The model under review builds one solid part; all positions refer to its coordinate system, in mm. Round coordinates to 2 decimals unless told otherwise and drop trailing zeros. Write each loop counter-clockwise with the first axis right and the second up, starting at its lowest first coordinate (ties: lowest second). Pieces come first, ordered by that corner, then holes. Notation, with made-up numbers: (49, -4.75) -> (59, -4.75) arc R13 ccw to (59, 12.25) -> close; hole circle Ø6 at (59.25, 44). An arc over 180 degrees is marked (long way). Return JSON: item names as keys, results as strings. Group by question number.
1. Take a section at A-A, the plane y = 0. Write out the cut boundary in (x, z), then the cut area to 3 significant figures.
2. For line 1 along Z through (x, y) = (7, 0); line 2 along Y through (x, z) = (20, 19.5); line 3 along Y through (x, z) = (7.5, -1), list the stretches that pass through material, from the lowest coordinate up. Write a range as from..to.
3. Clearance check with flat-ended pins moving along their axes: P1, Ø2, axis at y = 39.5, z = -31, coming from the +X side; P2, Ø10, axis at x = 20.5, z = -26, coming from the +Y side; P3, Ø5, axis at x = 3.5, y = 34.5, coming from the -Z side. State where each tip first meets the part, or that it passes through.
4. Mouldability with a two-part tool opening along Z and no side actions: class faces 1 (the cylindrical face through (14.79, -8.67, -39.05)), 2 (the flat face through (0, -18, 36)), 3 (the cylindrical face through (14.82, 47.69, 15.02)) as pulls with the +Z half, pulls with the -Z half, needs draft (parallel to the pull), parting line crosses it, or undercut.
5. Take a section at C-C, the plane x = 3.25. Write out the cut boundary in (y, z), then the cut area to 3 significant figures.
from build123d import *

# Parameters (mm, degrees)
F0_R     = 50
F0_R_2   = 40
F1_DEPTH = 28
F2_DEPTH = 30
F3_R     = 2
F4_R     = 2


with BuildPart() as f1:
    # F0 (on Right) → F1 (new body)
    with BuildSketch(Plane.YZ):
        Circle(F0_R)
        Circle(F0_R_2, mode=Mode.SUBTRACT)
    extrude(amount=F1_DEPTH)

    # F0 (on Right) → F2 (join)
    with BuildSketch(Plane.YZ):
        Circle(F0_R)
        Circle(F0_R_2, mode=Mode.SUBTRACT)
    extrude(amount=F2_DEPTH)

    # F3
    f3_edges = [f1.edges().sort_by_distance(p)[0] for p in [
        (30, -50, 0),
    ]]
    fillet(f3_edges, radius=F3_R)

    # F4
    f4_edges = [f1.edges().sort_by_distance(p)[0] for p in [
        (0, -50, 0),
    ]]
    fillet(f4_edges, radius=F4_R)


solid = f1.part
Output:
{
 "1": {"outline": "(0, -48) arc R2 ccw to (2, -50) -> (28, -50) arc R2 ccw to (30, -48) -> (30, -40) -> (0, -40) -> close; (0, 40) -> (30, 40) -> (30, 48) arc R2 ccw to (28, 50) -> (2, 50) arc R2 ccw to (0, 48) -> close", "area": "597 mm^2"},
 "2": {"line 1": "z = -50..-40, 40..50", "line 2": "y = -46.04..-34.92, 34.92..46.04", "line 3": "y = -49.99..-39.99, 39.99..49.99"},
 "3": {"P1": "stops at x = 29.59", "P2": "stops at y = 45.38", "P3": "stops at z = -38.42"},
 "4": {"face 1": "undercut", "face 2": "needs draft", "face 3": "parting line crosses it"},
 "5": {"outline": "circle Ø100 at (0, 0); hole circle Ø80 at (0, 0)", "area": "2,830 mm^2"}
}
